Drawing for the job (mm, zero at the part's lowest x, y, z). Coordinates: 2 decimals unless noted, no trailing zeros. Write each loop counter-clockwise with the first axis right and the second up, starting at its lowest first coordinate (ties: lowest second). Pieces come first, ordered by that corner, then holes. Notation, with made-up numbers: (72, 52.5) -> (128, 52.5) arc R19 ccw to (128, 76.5) -> close; hole circle Ø3 at (41.25, 85). An arc over 180 degrees is marked (long way). Write item = value, one per line. Start each with the question number.
Q1. Pin check, flat tips, straight feed: P1, Ø4.5, axis at x = 3, y = 5, coming from the +Z side; P2, Ø5.5, axis at y = 5, z = 6, coming from the -X side; P3, Ø4.5, axis at y = 68.5, z = 6, coming from the -X side. Stop position of each tip, or through.
Q2. Band-saw the part on B-B, the plane y = 5. List the corners of the cut face in (x, z), plus the area to 3 significant figures.
Q3. Band-saw the part on C-C, the plane x = 2.5. List the corners of the cut face in (y, z).
Q4. Band-saw the part on A-A, the plane z = 6. List the corners of the cut face in (x, y), plus the area to 3 significant figures.
Q5. Band-saw the part on D-D, the plane y = 76.5. List the corners of the cut face in (x, z), plus the area to 3 significant figures.
Q6. Probe line 1 (Y direction, x = 2.2, z = 6); line 2 (Y direction, x = 3, z = 11.2); line 3 (Z direction, x = 6.5, y = 76.5). List the from-to ranges inside material, lowest first.
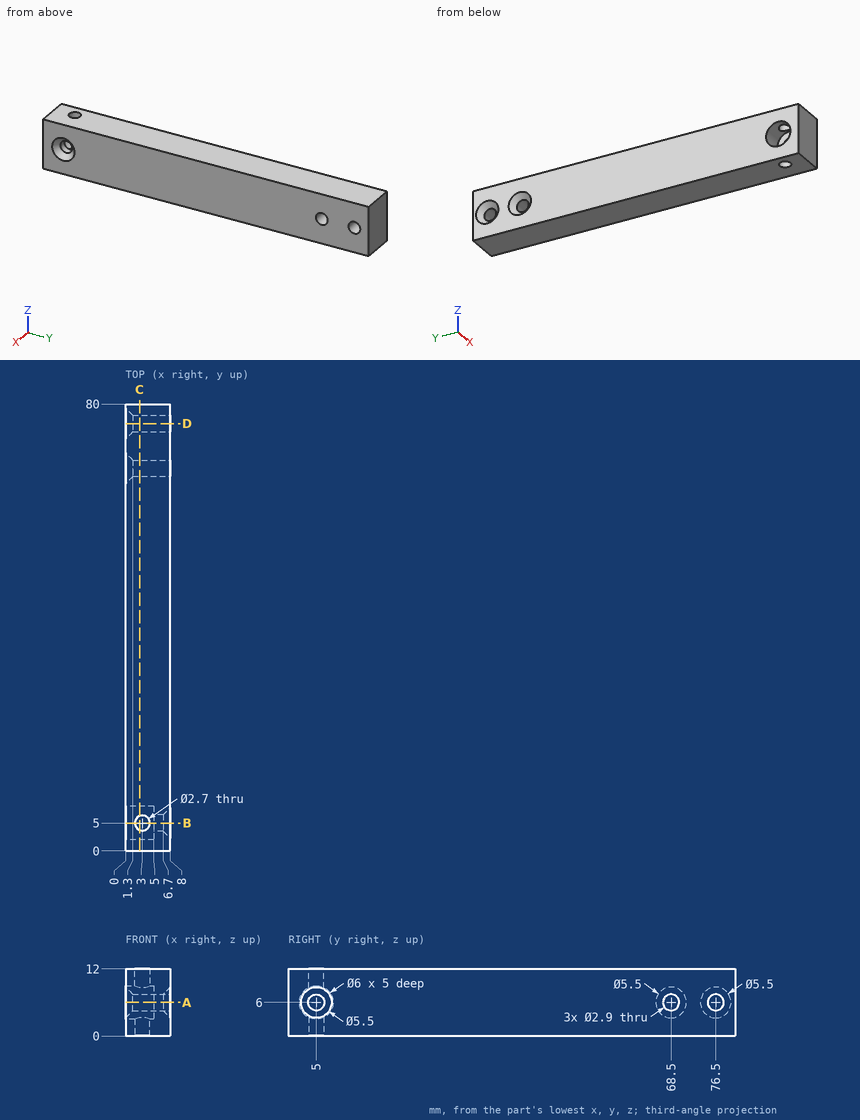
Ans:
q1.P1 = 12
q1.P2 = 5
q1.P3 = 0.5
q2.outline = (0, 0) -> (1.65, 0) -> (1.65, 3) -> (0, 3) -> close; (0, 9) -> (1.65, 9) -> (1.65, 12) -> (0, 12) -> close; (4.35, 0) -> (8, 0) -> (8, 3.25) -> (6.7, 4.55) -> (5, 4.55) -> (5, 3) -> (4.35, 3) -> close; (4.35, 9) -> (5, 9) -> (5, 7.45) -> (6.7, 7.45) -> (8, 8.75) -> (8, 12) -> (4.35, 12) -> close
q2.area = 39.4 mm2
q3.outline = (0, 0) -> (3.75, 0) -> (3.75, 3.27) arc R3 cw to (3.75, 8.73) -> (3.75, 12) -> (0, 12) -> close; (6.25, 0) -> (80, 0) -> (80, 12) -> (6.25, 12) -> (6.25, 8.73) arc R3 cw to (6.25, 3.27) -> close; hole circle Ø2.9 at (68.5, 6); hole circle Ø2.9 at (76.5, 6)
q4.outline = (0, 0) -> (8, 0) -> (8, 2.25) -> (6.7, 3.55) -> (5, 3.55) -> (5, 2) -> (0, 2) -> close; (0, 8) -> (5, 8) -> (5, 6.45) -> (6.7, 6.45) -> (8, 7.75) -> (8, 67.05) -> (1.3, 67.05) -> (0, 65.75) -> close; (0, 71.25) -> (1.3, 69.95) -> (8, 69.95) -> (8, 75.05) -> (1.3, 75.05) -> (0, 73.75) -> close; (0, 79.25) -> (1.3, 77.95) -> (8, 77.95) -> (8, 80) -> (0, 80) -> close
q4.area = 550 mm2
q5.outline = (0, 0) -> (8, 0) -> (8, 4.55) -> (1.3, 4.55) -> (0, 3.25) -> close; (0, 8.75) -> (1.3, 7.45) -> (8, 7.45) -> (8, 12) -> (0, 12) -> close
q5.area = 71.1 mm2
q6.line_1 = 0 to 2, 8 to 67.05, 69.95 to 75.05, 77.95 to 80
q6.line_2 = 0 to 3.65, 6.35 to 80
q6.line_3 = 0 to 4.55, 7.45 to 12
